Work out the finished part from the listing and answer in its coordinate system (mm). Give positions to 0.01 mm unless a question says otherwise; leave off trailing zeros. Order: outer loops, then holes, each group sorted by start corner. A loop starts at its lowest first (then second) coordinate and runs counter-clockwise, first axis right, second up. Notation, with made-up numbers: (-28, 40) - (12, 40) arc R24 cw to (12, 77) - close; hole circle Ø11 at (26.25, -4). An arc over 180 degrees is marked (long way). Write each question's results on one line, items separated by ' | '.
from build123d import *

# Parameters (mm, degrees)
PLAT_W                      = 160
PLAT_H                      = 10
EL_MENT_M_CANO_SOUD_1_DEPTH = 150
D_GAGEMENT_M161_D           = 17.5
D_GAGEMENT_M161_DEPTH       = 10
D_GAGEMENT_M161_TIP         = 5.257530416
ESQUISSE4_W                 = 10.5
ESQUISSE4_H                 = 10.5
ENL_V_MAT_EXTRU_1_DEPTH     = 11
CONG_1_R                    = 5
ENL_V_MAT_EXTRU_2_DEPTH     = 10


with BuildPart() as part:
    # plat → Elément mécano-soudé1 (new body)
    with BuildSketch(Plane.YZ):
        Rectangle(PLAT_W, PLAT_H)
    extrude(amount=EL_MENT_M_CANO_SOUD_1_DEPTH)

    # Dégagement M161
    with Locations(Plane.XY.offset(5)):
        with Locations((130, -60), (130, 60), (20, 60), (20, -60)):
            Hole(D_GAGEMENT_M161_D / 2, depth=D_GAGEMENT_M161_DEPTH)
            with Locations((0, 0, -(D_GAGEMENT_M161_DEPTH + D_GAGEMENT_M161_TIP / 2))):  # 118° drill point
                Cone(0, D_GAGEMENT_M161_D / 2, D_GAGEMENT_M161_TIP, mode=Mode.SUBTRACT)

    # Esquisse4 → Enlèv. mat.-Extru.1 (cut, through all)
    with BuildSketch(Plane.XY.offset(5)):
        with Locations((99.75, 74.75)):
            Rectangle(ESQUISSE4_W, ESQUISSE4_H)
        with Locations((99.75, -74.75)):
            Rectangle(ESQUISSE4_W, ESQUISSE4_H)
    extrude(amount=-ENL_V_MAT_EXTRU_1_DEPTH, mode=Mode.SUBTRACT)

    # Congé1
    cong_1_edges = [part.edges().sort_by_distance(p)[0] for p in [
        (150, 80, 0),
        (150, -80, 0),
        (0, 80, 0),
        (0, -80, 0),
    ]]
    fillet(cong_1_edges, radius=CONG_1_R)

    # Esquisse5 → Enlèv. mat.-Extru.2 (cut)
    with BuildSketch(Plane.XY.offset(5)):
        with BuildLine():
            Line((11.25, 56.5), (11.25, 63.5))
            ThreePointArc((11.25, 63.5), (20, 72.25), (28.75, 63.5))
            Line((28.75, 63.5), (28.75, 56.5))
            ThreePointArc((28.75, 56.5), (20, 47.75), (11.25, 56.5))
        make_face()
        with BuildLine():
            Line((138.75, 56.5), (138.75, 63.5))
            ThreePointArc((138.75, 63.5), (130, 72.25), (121.25, 63.5))
            Line((121.25, 63.5), (121.25, 56.5))
            ThreePointArc((121.25, 56.5), (130, 47.75), (138.75, 56.5))
        make_face()
        with BuildLine():
            Line((138.75, -56.5), (138.75, -63.5))
            ThreePointArc((138.75, -63.5), (130, -72.25), (121.25, -63.5))
            Line((121.25, -63.5), (121.25, -56.5))
            ThreePointArc((121.25, -56.5), (130, -47.75), (138.75, -56.5))
        make_face()
        with BuildLine():
            Line((11.25, -56.5), (11.25, -63.5))
            ThreePointArc((11.25, -63.5), (20, -72.25), (28.75, -63.5))
            Line((28.75, -63.5), (28.75, -56.5))
            ThreePointArc((28.75, -56.5), (20, -47.75), (11.25, -56.5))
        make_face()
    extrude(amount=-ENL_V_MAT_EXTRU_2_DEPTH, mode=Mode.SUBTRACT)


solid = part.part
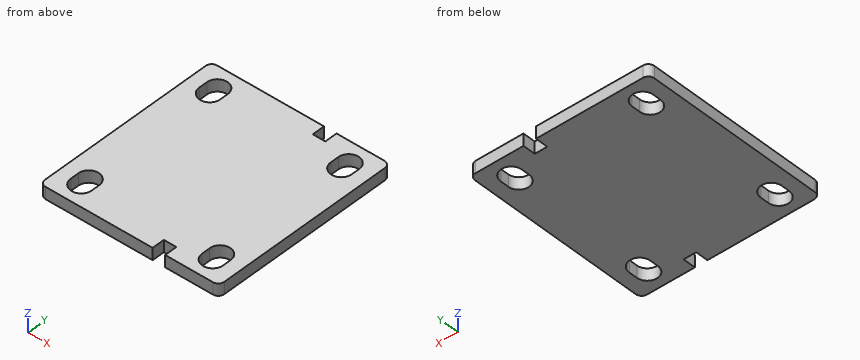
1. Straight lines are drawn through the part: line 1 (X direction, y = 60.5, z = -1.25); line 2 (Y direction, x = 126, z = 2); line 3 (X direction, y = -51, z = 1.5). For each, find the intervals that lie inside material, in ascending order. Write a range as [from, to].
Answer list:
line 1: [0, 11.25], [28.75, 121.25], [138.75, 150] | line 2: [-80, -71.28], [-48.72, 48.72], [71.28, 80] | line 3: [0, 13.19], [26.81, 123.19], [136.81, 150]
2. A cutting plane is placed at C-C, the plane z = -2.25. State how many separate pieces and enclosed holes the cut face has, then the cut area to 3 significant figures.
Answer list:
separate pieces: 1 | enclosed holes: 4 | area: 22,300 mm^2
3. A cutting plane is placed at A-A, the plane x = 130. Write down the section's boundary in (y, z), then the cut area to 3 significant figures.
Answer list:
outline: (-80, -5) - (-72.25, -5) - (-72.25, 5) - (-80, 5) - close; (-47.75, -5) - (47.75, -5) - (47.75, 5) - (-47.75, 5) - close; (72.25, -5) - (80, -5) - (80, 5) - (72.25, 5) - close | area: 1,110 mm^2
4. Given P1, Ø5, axis at x = 99.5, z = 1.5, coming from the +Y side; P2, Ø5, axis at x = 102, z = 0.5, coming from the -Y side, each flat-ended and moving along its own axis, determine where each tip first touches the part or whether it passes through.
Answer list:
P1: y = 69.5 | P2: y = -69.5
5. A cutting plane is placed at B-B, the plane y = 60. Write down the section's boundary in (x, z).
Answer list:
outline: (0, -5) - (11.25, -5) - (11.25, 5) - (0, 5) - close; (28.75, -5) - (121.25, -5) - (121.25, 5) - (28.75, 5) - close; (138.75, -5) - (150, -5) - (150, 5) - (138.75, 5) - close
